from build123d import *

# Parameters (mm, degrees)
F0_R     = 2.5
F1_DEPTH = 5


with BuildPart() as f1:
    # F0 (on Front) → F1 (new body)
    with BuildSketch(Plane.XZ):
        with BuildLine():
            Line((0, 97.928932), (0, 5))
            ThreePointArc((0, 5), (1.464466, 1.464466), (5, 0))
            Line((5, 0), (195, 0))
            ThreePointArc((195, 0), (198.535534, 1.464466), (200, 5))
            Line((200, 5), (200, 95))
            ThreePointArc((200, 95), (198.535534, 98.535534), (195, 100))
            Line((195, 100), (185, 100))
            ThreePointArc((185, 100), (181.464466, 101.464466), (180, 105))
            Line((180, 105), (180, 195))
            ThreePointArc((180, 195), (178.535534, 198.535534), (175, 200))
            Line((175, 200), (102.071068, 200))
            ThreePointArc((102.071068, 200), (100.157651, 199.619398), (98.535534, 198.535534))
            Line((98.535534, 198.535534), (1.464466, 101.464466))
            ThreePointArc((1.464466, 101.464466), (0.380602, 99.842349), (0, 97.928932))
        make_face()
        with Locations((25, 20)):
            Circle(F0_R, mode=Mode.SUBTRACT)
        with Locations((65, 20)):
            Circle(F0_R, mode=Mode.SUBTRACT)
        with Locations((25, 60)):
            Circle(F0_R, mode=Mode.SUBTRACT)
        with Locations((25, 80)):
            Circle(F0_R, mode=Mode.SUBTRACT)
        with Locations((65, 60)):
            Circle(F0_R, mode=Mode.SUBTRACT)
        with Locations((135.282773, 19.887757)):
            Circle(F0_R, mode=Mode.SUBTRACT)
        with Locations((175, 20)):
            Circle(F0_R, mode=Mode.SUBTRACT)
        with Locations((135, 60)):
            Circle(F0_R, mode=Mode.SUBTRACT)
        with Locations((100, 80)):
            Circle(F0_R, mode=Mode.SUBTRACT)
        with Locations((175, 60)):
            Circle(F0_R, mode=Mode.SUBTRACT)
        with Locations((175, 80)):
            Circle(F0_R, mode=Mode.SUBTRACT)
    extrude(amount=F1_DEPTH)


solid = f1.part
Verification items for the finished model (mm, model axes). Give positions to 0.01 mm unless a question says otherwise; leave off trailing zeros. Loops run counter-clockwise (first coordinate to the right, second up) from the corner with the lowest first, then second, coordinate; pieces in that order, holes last. Notation, with made-up numbers: (74, 37) - (82, 37) arc R22 ccw to (82, 48) - close; hole circle Ø11 at (17.25, 29). An arc over 180 degrees is marked (long way). Write item = value, one per line. Start each with the question number.
Q1. Cross-section at B-B, the plane y = -2.8. State how many separate pieces and enclosed holes the cut face has, and give its area (3 significant figures).
Q2. Depth check by flat-ended pin: P1, Ø4.5, axis at x = 100, z = 80, coming from the +Y side; P2, Ø3, axis at y = -3, z = 137, coming from the +X side. Enter the tip coordinate at first touch or a pass-through.
Q3. Cross-section at C-C, the plane x = 20. Enter the section's corners in (y, z).
Q4. Mould release check, pull along X, two halves, no side actions. Record for faces 1 (the face through (177.385, -2.465, 20.751)), 2 (the face through (99, 0, 101)), 3 (the face through (137.385, -2.465, 60.751)), 4 (the face through (0, -2, 52)): released by +X, released by -X, zero draft, split by the parting line, or undercut.
Q5. Cross-section at A-A, the plane x = 65. Enter the section's corners in (y, z).
Q6. Thickness scan on line 1 (Z direction, x = 175, y = -3.4); line 2 (Z direction, x = 66, y = -3.65); line 3 (Z direction, x = 65, y = -2.8). Record the ranges inside material, lowest first.
Answer key:
q1.separate_pieces = 1
q1.enclosed_holes = 11
q1.area = 32,800 mm^2
q2.P1 = through
q2.P2 = 180
q3.outline = (-5, 0) - (0, 0) - (0, 120) - (-5, 120) - close
q4.face_1 = undercut
q4.face_2 = zero draft
q4.face_3 = undercut
q4.face_4 = released by -X
q5.outline = (-5, 0) - (0, 0) - (0, 17.5) - (-5, 17.5) - close; (-5, 22.5) - (0, 22.5) - (0, 57.5) - (-5, 57.5) - close; (-5, 62.5) - (0, 62.5) - (0, 165) - (-5, 165) - close
q6.line_1 = 0 to 17.5, 22.5 to 57.5, 62.5 to 77.5, 82.5 to 200
q6.line_2 = 0 to 17.71, 22.29 to 57.71, 62.29 to 166
q6.line_3 = 0 to 17.5, 22.5 to 57.5, 62.5 to 165
